Autodesk Fusion 360 part; units mm, degrees
sketch "スケッチ1" plane through (0, 0, 0) normal (0, 1, 0) x (1, 0, 0)
  circle A0 centre (0, 0) radius 1.6
  circle A1 centre (0, 0) radius 5
  line L0 (0, 5) -> (30, 5)
  line L1 (30, 5) -> (30, -5)
  line L2 (30, -5) -> (0, -5)
  line L3 (0, -5) -> (0, 5)
  dimension "d1" = 3.2
  dimension "d2" = 30
  dimension "d3" = 10
extrude "押し出し1" add sketch "スケッチ1" along normal blind 3 contours A0 A1 L3 | A0 A1 L3 | A1 L0 L1 L2
sketch "スケッチ2" plane through (0, 3, 0) normal (0, 1, 0) x (-1, 0, 0)
  circle A0 centre (0, 0) radius 1.6
  arc A1 (0, -5) -> (0, 5) centre (0, 0) ccw
  line L0 (0, 5) -> (-30, 5)
  line L1 (-30, 5) -> (-30, -5)
  line L2 (-30, -5) -> (0, -5)
  line L3 (-30, -5) -> (-27, -5)
  line L4 (-27, -5) -> (-27, 5)
  line L5 (-27, 5) -> (-30, 5)
  line L6 (-30, 5) -> (-30, -5)
  dimension "d6" = 3
  dimension "d7" = 10
extrude "押し出し2" add sketch "スケッチ2" along normal blind 30 contours L0 L1 L2 L3 L4 L5 L6
sketch "スケッチ3" plane through (0, 33, 0) normal (0, 1, 0) x (-1, 0, 0)
  line L0 (-30, 5) -> (-30, -5)
  line L1 (-30, -5) -> (-27, -5)
  line L2 (-27, -5) -> (-27, 5)
  line L3 (-27, 5) -> (-30, 5)
  line L4 (-27, 5) -> (-27, -5)
  line L5 (-27, -5) -> (0, -5)
  arc A0 (0, -5) -> (0, 5) centre (0, 0) ccw
  line L6 (0, 5) -> (-27, 5)
  circle A1 centre (0, 0) radius 1.6
extrude "押し出し3" add sketch "スケッチ3" along normal blind 3
extrude "押し出し4" add 1 faces at (19.5096, 36, -0.1572) along direction (0, 1, 0) blind 3
extrude "押し出し5" cut 1 faces at (18.5333, 33, 0) along direction (0, 1, 0) blind 3
extrude "押し出し6" add 1 faces at (19.5096, 39, -0.1572) along direction (0, 1, 0) blind 2
extrude "押し出し7" cut 1 faces at (18.5333, 36, 0) along direction (0, 1, 0) blind 2
extrude "押し出し8" add 1 faces at (18.5333, 38, 0) along direction (0, -1, 0) blind 2
extrude "押し出し9" cut 1 faces at (19.5096, 41, -0.1572) along direction (0, -1, 0) blind 2
extrude "押し出し10" add 1 faces at (19.5096, 39, -0.1572) along direction (0, 1, 0) blind 1
sketch "スケッチ4" plane through (0, 40, 0) normal (0, 1, 0) x (-1, 0, 0)
  circle A0 centre (0, 0) radius 1.6
  line L0 (0, 5) -> (-30, 5)
  line L1 (-30, 5) -> (-30, -5)
  line L2 (-30, -5) -> (0, -5)
  arc A1 (0, -5) -> (0, 5) centre (0, 0) ccw
  circle A2 centre (0, 0) radius 3.6
  dimension "d26" = 7.2
extrude "押し出し11" cut sketch "スケッチ4" against normal blind 10 contours A2
sketch "スケッチ5" plane through (0, 40, 0) normal (0, 1, 0) x (-1, 0, 0)
  circle A0 centre (0, 0) radius 3.6
  line L0 (0, 5) -> (-30, 5)
  line L1 (-30, 5) -> (-30, -5)
  line L2 (-30, -5) -> (0, -5)
  arc A1 (0, -5) -> (0, 5) centre (0, 0) ccw
  circle A2 centre (0, 0) radius 3.6
  line L3 (0, 0) -> (-2.3505, 0)
  line L4 (-2.3505, 0) -> (-16.8505, 0)
  circle A3 centre (-16.8505, 0) radius 2.1
  line L5 (-17.0374, -2.0917) -> (-0.3205, -3.5857)
  line L6 (-17.0374, 2.0917) -> (-0.3205, 3.5857)
  dimension "d29" = 14.5
  dimension "d30" = 4.2
extrude "押し出し12" cut sketch "スケッチ5" against normal blind 2 contours A0 A2 L4 A3 L6 | A0 A2 L4 A3 L5 | A3
extrude "押し出し13" cut 1 faces at (18.5333, 3, 0) along direction (0, -1, 0) blind 2
extrude "押し出し14" add 1 faces at (20.5333, 0, 0) along direction (0, -1, 0) blind 2
sketch "スケッチ6" plane through (30, 0, 0) normal (1, 0, 0) x (0, 0, -1)
  line L0 (-5, 40) -> (-5, -2)
  line L1 (-5, -2) -> (5, -2)
  line L2 (5, -2) -> (5, 40)
  line L3 (5, 40) -> (-5, 40)
  line L4 (5, -2) -> (5, -1)
  line L5 (-5, 40) -> (5, -2)
  line L6 (12, 26.5) -> (-12, 26.5)
  line L7 (-12, 26.5) -> (-12, 11.5)
  line L8 (-12, 11.5) -> (12, 11.5)
  line L9 (12, 11.5) -> (12, 26.5)
  line L10 (12, 26.5) -> (-12, 11.5) construction
  line L11 (-12, 26.5) -> (12, 11.5) construction
  line L12 (-12, 26.5) -> (-9, 26.5)
  line L13 (-9, 26.5) -> (-9, 23.5)
  line L14 (-9, 23.5) -> (-12, 23.5)
  line L15 (-12, 23.5) -> (-12, 26.5)
  line L16 (-12, 11.5) -> (-9, 11.5)
  line L17 (-9, 11.5) -> (-9, 14.5)
  line L18 (-9, 14.5) -> (-12, 14.5)
  line L19 (-12, 14.5) -> (-12, 11.5)
  line L20 (12, 26.5) -> (9, 26.5)
  line L21 (9, 26.5) -> (9, 23.5)
  line L22 (9, 23.5) -> (12, 23.5)
  line L23 (12, 23.5) -> (12, 26.5)
  line L24 (12, 11.5) -> (9, 11.5)
  line L25 (9, 11.5) -> (9, 14.5)
  line L26 (9, 14.5) -> (12, 14.5)
  line L27 (12, 14.5) -> (12, 11.5)
  circle A0 centre (-9, 23.5) radius 1.6
  circle A1 centre (-9, 14.5) radius 1.6
  circle A2 centre (9, 14.5) radius 1.6
  circle A3 centre (9, 23.5) radius 1.6
  point P0 (0, 19)
  dimension "d37" = 24
  dimension "d38" = 15
  dimension "d39" = 3
  dimension "d40" = 3
  dimension "d41" = 3
  dimension "d42" = 3
  dimension "d43" = 3
  dimension "d44" = 3
  dimension "d45" = 3
  dimension "d46" = 3
  dimension "d47" = 3.2
  dimension "d48" = 3.2
  dimension "d49" = 3.2
  dimension "d50" = 3.2
extrude "押し出し15" add sketch "スケッチ6" against normal blind 3 contours L0 L6 L7 L8 L13 L14 L17 L18 A0 A1 | L6 L7 L12 L13 L14 L15 A0 | L2 L6 L8 L9 L21 L22 L25 L26 A2 A3 | L7 L8 L16 L17 L18 L19 A1 | L6 L9 L20 L21 L22 L23 A3 | L8 L9 L24 L25 L26 L27 A2
chamfer "面取り1" distance 2 angle 45 4 edges at (28.5, 11.5, -12) (28.5, 26.5, -12) (28.5, 26.5, 12) (28.5, 11.5, 12)
sketch "スケッチ7" plane through (30, 0, 0) normal (1, 0, 0) x (0, 0, -1)
  circle A0 centre (-9, 14.5) radius 1.6
  circle A1 centre (-9, 23.5) radius 1.6
  circle A2 centre (9, 23.5) radius 1.6
  circle A3 centre (9, 14.5) radius 1.6
  line L0 (-12, 13.5) -> (-10, 11.5)
  line L1 (-10, 11.5) -> (-5, 11.5)
  line L2 (-5, 11.5) -> (-5, -2)
  line L3 (-5, -2) -> (5, -2)
  line L4 (5, -2) -> (5, 11.5)
  line L5 (5, 11.5) -> (10, 11.5)
  line L6 (10, 11.5) -> (12, 13.5)
  line L7 (12, 13.5) -> (12, 24.5)
  line L8 (12, 24.5) -> (10, 26.5)
  line L9 (10, 26.5) -> (5, 26.5)
  line L10 (5, 26.5) -> (5, 40)
  line L11 (5, 40) -> (-5, 40)
  line L12 (-5, 40) -> (-5, 26.5)
  line L13 (-5, 26.5) -> (-10, 26.5)
  line L14 (-10, 26.5) -> (-12, 24.5)
  line L15 (-12, 24.5) -> (-12, 13.5)
  line L16 (-12, 19) -> (12, 19)
  line L17 (0, 19) -> (0, 15.95)
  line L18 (0, 15.95) -> (4, 15.95)
  line L19 (0, 15.95) -> (-4, 15.95)
  line L20 (-4, 15.95) -> (4, 15.95)
  line L21 (4, 15.95) -> (4, 10.95)
  line L22 (4, 10.95) -> (-4, 10.95)
  line L23 (-4, 10.95) -> (-4, 15.95)
  line L24 (-4, 15.95) -> (-4, 22.05)
  line L25 (-4, 22.05) -> (4, 22.05)
  line L26 (4, 22.05) -> (4, 27.05)
  line L27 (4, 27.05) -> (-4, 27.05)
  line L28 (-4, 27.05) -> (-4, 22.05)
  dimension "d54" = 3.05
  dimension "d55" = 4
  dimension "d56" = 4
  dimension "d57" = 8
  dimension "d58" = 5
  dimension "d59" = 6.1
  dimension "d60" = 8
  dimension "d61" = 5
extrude "押し出し16" cut sketch "スケッチ7" against normal blind 11 contours L25 L26 L27 L28 | L18 L19 L20 L21 L22 L23
chamfer "面取り2" distance 2 angle 45 4 edges at (28.5, 26.5, 5) (28.5, 26.5, -5) (28.5, 11.5, -5) (28.5, 11.5, 5)
extrude "押し出し17" cut 1 faces at (27, 4.5, -1.6667) along direction (1, 0, 0) blind 1
extrude "押し出し18" add 1 faces at (30, 3.5, -1.6667) along direction (1, 0, 0) blind 1
sketch "スケッチ8" plane through (31, 0, 0) normal (1, 0, 0) x (0, 0, -1)
  line L0 (4, 22.05) -> (-4, 22.05)
  line L1 (-4, 22.05) -> (-4, 27.05)
  line L2 (-4, 27.05) -> (4, 27.05)
  line L3 (4, 27.05) -> (4, 22.05)
  line L4 (4, 15.95) -> (4, 10.95)
  line L5 (4, 10.95) -> (-4, 10.95)
  line L6 (-4, 10.95) -> (-4, 15.95)
  line L7 (-4, 15.95) -> (4, 15.95)
  circle A0 centre (-9, 14.5) radius 1.6
  circle A1 centre (-9, 23.5) radius 1.6
  circle A2 centre (9, 23.5) radius 1.6
  circle A3 centre (9, 14.5) radius 1.6
  line L8 (-12, 13.5) -> (-10, 11.5)
  line L9 (-10, 11.5) -> (-7, 11.5)
  line L10 (-7, 11.5) -> (-5, 9.5)
  line L11 (-5, 9.5) -> (-5, -2)
  line L12 (-5, -2) -> (5, -2)
  line L13 (5, -2) -> (5, 9.5)
  line L14 (5, 9.5) -> (7, 11.5)
  line L15 (7, 11.5) -> (10, 11.5)
  line L16 (10, 11.5) -> (12, 13.5)
  line L17 (12, 13.5) -> (12, 24.5)
  line L18 (12, 24.5) -> (10, 26.5)
  line L19 (10, 26.5) -> (7, 26.5)
  line L20 (7, 26.5) -> (5, 28.5)
  line L21 (5, 28.5) -> (5, 40)
  line L22 (5, 40) -> (-5, 40)
  line L23 (-5, 40) -> (-5, 28.5)
  line L24 (-5, 28.5) -> (-7, 26.5)
  line L25 (-7, 26.5) -> (-10, 26.5)
  line L26 (-10, 26.5) -> (-12, 24.5)
  line L27 (-12, 24.5) -> (-12, 13.5)
  line L28 (-5, 28.5) -> (-5, 9.5)
  line L29 (5, 28.5) -> (5, 9.5)
extrude "押し出し19" cut sketch "スケッチ8" against normal blind 10 contours L8 L9 L10 L24 L25 L26 L27 L28 | L14 L15 L16 L17 L18 L19 L20 L29
sketch "スケッチ9" plane through (31, 0, 0) normal (1, 0, 0) x (0, 0, -1)
  line L0 (-5, 40) -> (-5, -2)
  line L1 (-5, -2) -> (5, -2)
  line L2 (5, -2) -> (5, 40)
  line L3 (5, 40) -> (-5, 40)
  line L4 (4, 22.05) -> (-4, 22.05)
  line L5 (-4, 22.05) -> (-4, 27.05)
  line L6 (-4, 27.05) -> (4, 27.05)
  line L7 (4, 27.05) -> (4, 22.05)
  line L8 (4, 15.95) -> (4, 10.95)
  line L9 (4, 10.95) -> (-4, 10.95)
  line L10 (-4, 10.95) -> (-4, 15.95)
  line L11 (-4, 15.95) -> (4, 15.95)
  line L12 (-4, 27.05) -> (4, 27.05)
  line L13 (4, 27.05) -> (4, 22.05)
  line L14 (4, 22.05) -> (-4, 22.05)
  line L15 (-4, 22.05) -> (-4, 27.05)
  line L16 (-4, 15.95) -> (4, 15.95)
  line L17 (4, 15.95) -> (4, 10.95)
  line L18 (4, 10.95) -> (-4, 10.95)
  line L19 (-4, 10.95) -> (-4, 15.95)
extrude "押し出し20" add sketch "スケッチ9" against normal blind 3 contours L4 L5 L6 L7 L12 L13 L14 L15 | L8 L9 L10 L11 L16 L17 L18 L19
sketch "スケッチ10" plane through (31, 0, 0) normal (1, 0, 0) x (0, 0, -1)
  line L0 (-5, 40) -> (-5, -2)
  line L1 (-5, -2) -> (5, -2)
  line L2 (5, -2) -> (5, 40)
  line L3 (5, 40) -> (-5, 40)
  line L4 (-5, 40) -> (5, -2)
  line L5 (4.5, 28) -> (-4.5, 28)
  line L6 (-4.5, 28) -> (-4.5, 10)
  line L7 (-4.5, 10) -> (4.5, 10)
  line L8 (4.5, 10) -> (4.5, 28)
  line L9 (4.5, 28) -> (-4.5, 10) construction
  line L10 (-4.5, 28) -> (4.5, 10) construction
  circle A0 centre (-4.5, 28) radius 1.6
  circle A1 centre (4.5, 28) radius 1.6
  circle A2 centre (-4.5, 10) radius 1.6
  circle A3 centre (4.5, 10) radius 1.6
  line L11 (-4.5, 28) -> (-7.3284, 30.8284)
  line L12 (-4.5, 28) -> (-0.5, 28) construction
  line L13 (-7.3284, 30.8284) -> (-5, 33.1569)
  line L14 (-4.5, 28) -> (-12, 28)
  line L15 (-7.3284, 30.8284) -> (-10.1569, 28)
  line L16 (-5, 33.1569) -> (-7.9773, 28)
  line L17 (-5, 33.1569) -> (0.9546, 33.1569) construction
  line L18 (-4.5, 10) -> (-11, 10)
  line L19 (-7.9773, 28) -> (-7.9773, 10)
  line L20 (-7.9773, 10) -> (-5, 4.8431)
  line L21 (-7.9773, 10) -> (-2.0227, 10) construction
  line L22 (4.5, 10) -> (11, 10)
  line L23 (0, 19) -> (0, 15)
  line L24 (5, 33.1569) -> (7.9773, 28)
  line L25 (7.9773, 28) -> (7.9773, 10)
  line L26 (7.9773, 10) -> (5, 4.8431)
  point P0 (0, 19)
  dimension "d73" = 9
  dimension "d74" = 18
  dimension "d75" = 3.2
  dimension "d76" = 3.2
  dimension "d77" = 3.2
  dimension "d78" = 3.2
  dimension "d79" = 135
  dimension "d80" = 4
  dimension "d81" = 120
  dimension "d82" = 60
extrude "押し出し21" add sketch "スケッチ10" against normal blind 3 contours L0 A0 L11 L16 | A0 L11 L14 L16 | L2 A1 A3 L22 L24 L25 | L0 A0 A2 L14 L18 L19 | L0 A2 L18 L20 | L2 A3 L22 L26
extrude "押し出し22" cut sketch "スケッチ10" against normal blind 3.5 contours L0 L5 A0 L11 | L2 L5 L8 A1 | L5 L8 A1 | L5 L6 A0 | L0 L11 L14 | L0 L6 A0 L14 | L0 L7 A2 L18 | L6 L7 A2 | L7 L8 A3 | L2 L7 A3 L22 | L2 L8 A3 L22 | L0 L6 A2 L18
For this review, take the finished solid that the model builds, in its own axes (mm). A direction names the side the tool comes from. Give positions to 0.01 mm unless a question says otherwise; leave off trailing zeros. Write each loop counter-clockwise with the first axis right and the second up, starting at its lowest first coordinate (ties: lowest second). Pieces come first, ordered by that corner, then holes. Notation, with made-up numbers: (14.5, 2) -> (69.5, 2) arc R24 cw to (69.5, 28) -> close; hole circle Ø11 at (-31, 78). An arc over 180 degrees is marked (long way). Use CSV: the item, a comma, the result in double quotes.
Q1. Mouldability with a two-part tool opening along X and no side actions: class faces 1 (the face through (-5, 0, 0)), 2 (the face through (31, 19, 0)), 3 (the face through (29.52, 26.46, 4.07)), 4 (the face through (8.796, 39.014, 2.828)) as pulls with the +X half, pulls with the -X half, needs draft (parallel to the pull), parting line crosses it, or undercut.
Conclusion:
face 1,"pulls with the -X half"
face 2,"pulls with the +X half"
face 3,"needs draft"
face 4,"undercut"
Q2. Tool access review of faces 5 (the face through (15, 0, 5)), 6 (the face through (18.95, 39.01, 0.04)), 7 (the face through (15, 0, -5)), 8 (the face through (11, 1, 0)): name each direction out of +Z, -Z, +X, -X, +Y, -Y from which nothing blocks a thin tool from reaching the whole face with its end or side.
Conclusion:
face 5,"+Z, +X, -X, -Y"
face 6,"+Y"
face 7,"-Z, +X, -X, -Y"
face 8,"+Z, -Z, -X"
Q3. For P1, Ø1.5, axis at y = 10.5, z = -5, coming from the -X side; P2, Ø7.5, axis at x = 22.5, y = 1, coming from the +Z side; P3, Ø5, axis at y = 32.5, z = -3, coming from the -X side; P4, Ø2, axis at x = 18.5, y = 37.5, coming from the -Z side, all flat-tipped, find the tip position at first contact; note any pin that passes through.
Conclusion:
P1,"through"
P2,"z = 5"
P3,"x = 28"
P4,"z = -5"
Q4. Take a section at B-B, the plane x = 25.5. Write out the cut boundary in (y, z), then the cut area to 3 significant figures.
Conclusion:
outline,"(-2, -5) -> (1, -5) -> (1, 5) -> (-2, 5) -> close; (36, -5) -> (40, -5) -> (40, 5) -> (36, 5) -> close"
area,"70.0 mm2"
Q5. To check wall thickness, follow probe 1 along Z at (x, y) = (29.95, 10); probe 2 along Y at (x, z) = (-0.5, -4.5); probe 3 along X at (y, z) = (38.95, 0). State the ranges of each line that lie inside material, in increasing order. Write a range as [from, to].
Conclusion:
probe 1,"[-7.98, -6.1], [-2.9, 2.9], [6.1, 7.98]"
probe 2,"[-2, 1], [36, 40]"
probe 3,"[-5, -3.6], [18.95, 31]"
Q6. Take a section at D-D, the plane y = 2.5. Write out the cut boundary in (x, z).
Conclusion:
outline,"(28, -5) -> (31, -5) -> (31, 5) -> (28, 5) -> close"
Q7. Take a section at C-C, the plane z = 4.25. Write out the cut boundary in (x, y), then the cut area to 3 significant figures.
Conclusion:
outline,"(-2.63, -2) -> (31, -2) -> (31, 8.42) -> (28, 8.42) -> (28, 1) -> (-2.63, 1) -> close; (-2.63, 36) -> (28, 36) -> (28, 29.58) -> (31, 29.58) -> (31, 40) -> (-2.63, 40) -> close; (28, 11.58) -> (31, 11.58) -> (31, 26.42) -> (28, 26.42) -> close"
area,"321 mm2"
Q8. Take a section at A-A, the plane z = 0. Write out the cut boundary in (x, y), then the cut area to 3 significant figures.
Conclusion:
outline,"(-5, -2) -> (-1.6, -2) -> (-1.6, 1) -> (-5, 1) -> close; (-5, 36) -> (-3.6, 36) -> (-3.6, 40) -> (-5, 40) -> close; (1.6, -2) -> (31, -2) -> (31, 40) -> (18.95, 40) -> (18.95, 38) -> (3.6, 38) -> (3.6, 36) -> (28, 36) -> (28, 1) -> (1.6, 1) -> close"
area,"288 mm2"
